```python
from build123d import *

# Parameters (mm, degrees)
F1_W           = 82.55
F1_H           = 66.675
F2_DEPTH       = 6.35
F4_D           = 11.303
F4_CBORE_D     = 21.717
F4_CBORE_DEPTH = 3.302
F6_D           = 6.985
F7_D           = 6.985
F8_D           = 5.207
F9_R           = 6.35
F11_D          = 5.207


with BuildPart() as f2:
    # F1 (on Top) → F2 (new body)
    with BuildSketch(Plane.XY):
        with Locations((0, 2.2225)):
            Rectangle(F1_W, F1_H)
    extrude(amount=F2_DEPTH)

    # F4 (through all)
    with Locations(Plane.XY.offset(6.35)):
        with Locations((0, 0)):
            CounterBoreHole(F4_D / 2, F4_CBORE_D / 2, F4_CBORE_DEPTH)

    # F6 (through all)
    with Locations(Plane.XY.offset(6.35)):
        with Locations((-27.2669, 26.4414)):
            Hole(F6_D / 2)

    # F7 (through all)
    with Locations(Plane.XY.offset(6.35)):
        with Locations((27.26436, 26.4414)):
            Hole(F7_D / 2)

    # F8 (through all)
    with Locations(Plane(origin=(0, 0, 0), x_dir=(1, 0, 0), z_dir=(0, 0, -1))):
        with Locations((23.622, 23.622), (-23.622, 23.622)):
            Hole(F8_D / 2)

    # F9
    f9_edges = [f2.edges().sort_by_distance(p)[0] for p in [
        (-41.275, -31.115, 3.175),
        (41.275, -31.115, 3.175),
        (41.275, 35.56, 3.175),
        (-41.275, 35.56, 3.175),
    ]]
    fillet(f9_edges, radius=F9_R)

    # F11 (through all)
    with Locations(Plane(origin=(0, 0, 0), x_dir=(1, 0, 0), z_dir=(0, 0, -1))):
        with Locations((-31.75, -11.43), (31.75, -11.43)):
            Hole(F11_D / 2)


solid = f2.part
```
For this review, take the finished solid that the model builds, in its own axes (mm). A direction names the side the tool comes from. Coordinates: 2 decimals unless noted, no trailing zeros. Write each loop counter-clockwise with the first axis right and the second up, starting at its lowest first coordinate (ties: lowest second). Pieces come first, ordered by that corner, then holes.
(1) Add section C-C on y = 3.5. Give the boundary of the cut face in (x, z) (3 decimals).
(2) Add section B-B on z = 1.25. Count the separate pieces of the cut face and the enclosed holes in it, then the cut area to 3 significant figures.
(3) The part is to be moulded in two halves that separate along Y. For faces 3 (the face through (-1, 10, 0)), 4 (the face through (-21.556, -22.038, 3.219)), 5 (the face through (-2.35, -10.6, 4.72)), 6 (the face through (39.37, -29.3, 3.22)), say which applies: +Y half, -Y half, draft (parallel to the pull), parting line (faces both ways), or undercut.
(4) Add section A-A on x = -2. Give the boundary of the cut face in (y, z) (3 decimals).
(5) For pin 1 Ø4 at (x, y) = (27, -21.5) entering from -Z; pin 2 Ø13 at (x, y) = (0, 0) entering from +Z, all flat-tipped, find the tip position at first contact; note any pin that passes through.
(6) Wall thickness on probe 1 along X at (y, z) = (-23.5, 4) (3 decimals); probe 2 along X at (y, z) = (-24.5, 1.5) (3 decimals); probe 3 along X at (y, z) = (5, 1.5) (3 decimals): over which ranges is each line inside the solid? List them lowest first.
(7) Tool access review of faces 1 (the face through (5, -5, 3.048)), 2 (the face through (-5.39, 1.7, 1.5)): name each direction out of +Z, -Z, +X, -X, +Y, -Y from which nothing blocks a thin tool from reaching the whole face with its end or side.
Answer sheet:
1. outline: (-41.275, 0) - (-4.437, 0) - (-4.437, 3.048) - (-10.279, 3.048) - (-10.279, 6.35) - (-41.275, 6.35) - close; (4.437, 0) - (41.275, 0) - (41.275, 6.35) - (10.279, 6.35) - (10.279, 3.048) - (4.437, 3.048) - close
2. separate pieces: 1
2. enclosed holes: 7
2. area: 5,210 mm2
3. face 3: draft
3. face 4: undercut
3. face 5: undercut
3. face 6: -Y half
4. outline: (-31.115, 0) - (-5.286, 0) - (-5.286, 3.048) - (-10.673, 3.048) - (-10.673, 6.35) - (-31.115, 6.35) - close; (5.286, 0) - (35.56, 0) - (35.56, 6.35) - (10.673, 6.35) - (10.673, 3.048) - (5.286, 3.048) - close
5. pin 1: stops at z = 0
5. pin 2: stops at z = 3.05
6. probe 1: x = -41.275 to -26.223, -21.021 to 21.021, 26.223 to 41.275
6. probe 2: x = -41.275 to -26.073, -21.171 to 21.171, 26.073 to 41.275
6. probe 3: x = -41.275 to -2.634, 2.634 to 41.275
7. face 1: +Z
7. face 2: +Z, -Z
